from build123d import *

# Parameters (mm, degrees)
SKETCH1_W           = 60.5
SKETCH1_H           = 38.5
BOSS_EXTRUDE1_DEPTH = 6
BOSS_EXTRUDE2_DEPTH = 4
SKETCH4_W           = 6
SKETCH4_H           = 19.5
BOSS_EXTRUDE4_DEPTH = 2
SKETCH6_R           = 2
CUT_EXTRUDE1_DEPTH  = 9
SKETCH7_W           = 48.5
SKETCH7_H           = 2.5
CUT_EXTRUDE2_DEPTH  = 2
CUT_EXTRUDE3_DEPTH  = 4.5
CUT_EXTRUDE4_DEPTH  = 3
SKETCH10_W          = 6
SKETCH10_H          = 7.5
CUT_EXTRUDE5_DEPTH  = 2
SKETCH13_W          = 6
SKETCH13_H          = 10
CUT_EXTRUDE6_DEPTH  = 1.5
CUT_EXTRUDE7_REACH  = 10
SKETCH14_R          = 2


with BuildPart() as part:
    # Sketch1 → Boss-Extrude1 (new body)
    with BuildSketch(Plane(origin=(0, 0, 0), x_dir=(1, 0, 0), z_dir=(0, 1, 0))):
        with Locations((6.235680191, -0.331443914)):
            Rectangle(SKETCH1_W, SKETCH1_H)
    extrude(amount=BOSS_EXTRUDE1_DEPTH)

    # Sketch2 → Boss-Extrude2 (add)
    with BuildSketch(Plane(origin=(0, 6, 0), x_dir=(1, 0, 0), z_dir=(0, 1, 0))):
        Polygon((-24.014319809, -19.581443914), (36.485680191, -19.581443914), (36.485680191, -14.581443914), (36.485680191, -7.081443914), (30.485680191, -7.081443914), (30.485680191, -14.581443914), (-18.014319809, -14.581443914), (-18.014319809, -8.581443914), (-24.014319809, -8.581443914), (-24.014319809, -14.581443914), align=None)
        Polygon((-24.014319809, 18.918556086), (36.485680191, 18.918556086), (36.485680191, 13.918556086), (36.485680191, 6.418556086), (30.485680191, 6.418556086), (30.485680191, 13.918556086), (-24.014319809, 13.918556086), align=None)
    extrude(amount=BOSS_EXTRUDE2_DEPTH)

    # Sketch4 → Boss-Extrude4 (add)
    with BuildSketch(Plane(origin=(0, 6, 0), x_dir=(1, 0, 0), z_dir=(0, 1, 0))):
        with Locations((-21.014319809, 4.168556086)):
            Rectangle(SKETCH4_W, SKETCH4_H)
    extrude(amount=BOSS_EXTRUDE4_DEPTH)

    # Sketch6 → Cut-Extrude1 (cut, through all)
    with BuildSketch(Plane(origin=(0, 8, 0), x_dir=(1, 0, 0), z_dir=(0, 1, 0))):
        with Locations((-21.014319809, -0.331443914)):
            Circle(SKETCH6_R)
    extrude(amount=-CUT_EXTRUDE1_DEPTH, mode=Mode.SUBTRACT)

    # Sketch7 → Cut-Extrude2 (cut)
    with BuildSketch(Plane(origin=(0, 6, 0), x_dir=(1, 0, 0), z_dir=(0, 1, 0))):
        with Locations((6.235680191, 12.668556086)):
            Rectangle(SKETCH7_W, SKETCH7_H)
        with Locations((6.235680191, -13.331443914)):
            Rectangle(SKETCH7_W, SKETCH7_H)
    extrude(amount=-CUT_EXTRUDE2_DEPTH, mode=Mode.SUBTRACT)

    # Sketch8 → Cut-Extrude3 (cut)
    with BuildSketch(Plane(origin=(0, 6, 0), x_dir=(1, 0, 0), z_dir=(0, 1, 0))):
        Polygon((-18.014319809, -5.581443914), (-18.014319809, 9.168556086), (2.985680191, 9.168556086), (2.985680191, -8.581443914), (2.985680191, -9.831443914), (-18.014319809, -9.831443914), (-18.014319809, -8.581443914), (-24.014319809, -8.581443914), (-24.014319809, -5.581443914), align=None)
    extrude(amount=-CUT_EXTRUDE3_DEPTH, mode=Mode.SUBTRACT)

    # Sketch9 → Cut-Extrude4 (cut)
    with BuildSketch(Plane(origin=(0, 6, 0), x_dir=(1, 0, 0), z_dir=(0, 1, 0))):
        Polygon((30.485680191, 9.918556086), (6.485680191, 9.918556086), (6.485680191, -9.581443914), (30.485680191, -9.581443914), (30.485680191, -7.081443914), (36.485680191, -7.081443914), (36.485680191, 6.418556086), (30.485680191, 6.418556086), align=None)
    extrude(amount=-CUT_EXTRUDE4_DEPTH, mode=Mode.SUBTRACT)

    # Sketch10 → Cut-Extrude5 (cut)
    with BuildSketch(Plane(origin=(0, 10, 0), x_dir=(1, 0, 0), z_dir=(0, 1, 0))):
        with Locations((33.485680191, 10.168556086)):
            Rectangle(SKETCH10_W, SKETCH10_H)
        with Locations((33.485680191, -10.831443914)):
            Rectangle(SKETCH10_W, SKETCH10_H)
    extrude(amount=-CUT_EXTRUDE5_DEPTH, mode=Mode.SUBTRACT)

    # Sketch13 → Cut-Extrude6 (cut)
    with BuildSketch(Plane(origin=(0, 3, 0), x_dir=(1, 0, 0), z_dir=(0, 1, 0))):
        with Locations((33.485680191, -0.331443914)):
            Rectangle(SKETCH13_W, SKETCH13_H)
    extrude(amount=-CUT_EXTRUDE6_DEPTH, mode=Mode.SUBTRACT)

    # Sketch14 → Cut-Extrude7 (cut, up to next)
    with BuildSketch(Plane(origin=(0, 8, 0), x_dir=(1, 0, 0), z_dir=(0, 1, 0)), mode=Mode.PRIVATE) as cut_extrude7_sk1:
        with Locations((33.485680191, -10.831443914)):
            Circle(SKETCH14_R)
    cut_extrude7_tool1 = extrude(cut_extrude7_sk1.sketch, amount=-CUT_EXTRUDE7_REACH, mode=Mode.PRIVATE) & part.part
    add(cut_extrude7_tool1.solids().sort_by_distance((33.48568, 8, 10.831444))[0], mode=Mode.SUBTRACT)
    # Sketch14 → Cut-Extrude7 (cut, up to next)
    with BuildSketch(Plane(origin=(0, 8, 0), x_dir=(1, 0, 0), z_dir=(0, 1, 0)), mode=Mode.PRIVATE) as cut_extrude7_sk2:
        with Locations((33.485680191, 10.168556086)):
            Circle(SKETCH14_R)
    cut_extrude7_tool2 = extrude(cut_extrude7_sk2.sketch, amount=-CUT_EXTRUDE7_REACH, mode=Mode.PRIVATE) & part.part
    add(cut_extrude7_tool2.solids().sort_by_distance((33.48568, 8, -10.168556))[0], mode=Mode.SUBTRACT)


solid = part.part
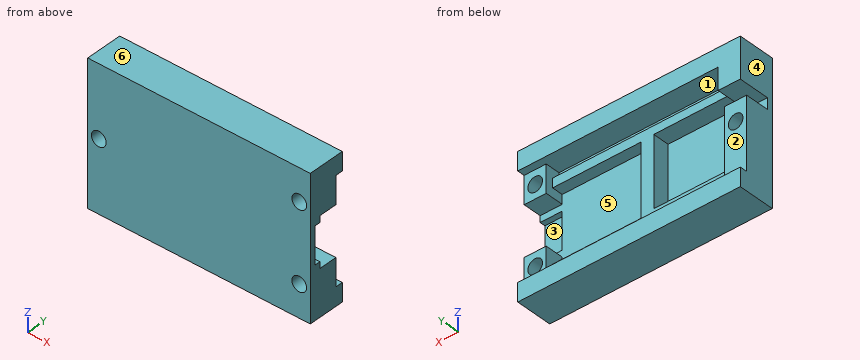
Geometry: final body of the model. Coordinates: model frame, mm. Face numbers are marked on the shaded views. A direction names the side the tool comes from. Round coordinates to 2 decimals unless told otherwise and drop trailing zeros. Write each loop counter-clockwise with the first axis right and the second up, starting at its lowest first coordinate (ties: lowest second). Pieces come first, ordered by that corner, then holes. Notation, with made-up numbers: M -29,-37 L -13,-37 A19 ccw -13,-7 Z; hole C 60.5,39.5 d7. An arc over 180 degrees is marked long. Write item = value, one per line.
Item 1: Pin query (flat end, axial travel): P1, Ø15, axis at x = -15.5, z = 3, coming from the +Y side; P2, Ø6, axis at x = 19, z = -4.5, coming from the +Y side; P3, Ø6, axis at x = -7, z = -2, coming from the +Y side; P4, Ø6.5, axis at x = 33.5, z = 9.5, coming from the +Y side. Return the tip coordinate at first contact, or that it passes through.
Findings:
P1 = 10
P2 = 3
P3 = 1.5
P4 = 8
Item 2: Access query for the marked faces 1, 2 and 3. Directions: +Z, -Z, +X, -X, +Y, -Y. A direction counts if a zero-diameter tool reaches every point of the face in a straight line with its end or side. Return the directions, or none.
Findings:
face_1 = +Y
face_2 = +X, -X, +Y
face_3 = +X, +Y
Item 3: Section query C-C on x = 20.5. Return loops of the section in (y, z).
Findings:
outline = M 0,-18.92 L 10,-18.92 L 10,-13.92 L 4,-13.92 L 4,-11.42 L 6,-11.42 L 6,-9.92 L 3,-9.92 L 3,9.58 L 6,9.58 L 6,12.08 L 4,12.08 L 4,14.58 L 10,14.58 L 10,19.58 L 0,19.58 Z
Item 4: Material intervals for line 1 along Z through (x, y) = (30, 6.5); line 2 along X through (y, z) = (1.5, 11); line 3 along Z through (x, y) = (14, 3.25), sorted ascending. Write a range as [from, to].
Findings:
line_1 = [-18.92, -13.92], [14.58, 19.58]
line_2 = [-24.01, 31.49], [35.48, 36.49]
line_3 = [-18.92, -9.92], [9.58, 19.58]
Item 5: Section query D-D on z = 8. Return loops of the section in (x, y).
Findings:
outline = M -24.01,0 L 36.49,0 L 36.49,8 L 30.49,8 L 30.49,3 L 6.49,3 L 6.49,6 L 2.99,6 L 2.99,1.5 L -24.01,1.5 Z
Item 6: Pull-direction query (X, two-part tool) for the marked faces 4, 5 and 6; classes: pulls with the +X half, pulls with the -X half, needs draft (parallel to the pull), parting line crosses it, or undercut.
Findings:
face_4 = pulls with the -X half
face_5 = undercut
face_6 = needs draft
Item 7: Section query A-A on y = 9. Return loops of the section in (x, z).
Findings:
outline = M -24.01,-18.92 L 36.49,-18.92 L 36.49,-13.92 L -24.01,-13.92 Z; M -24.01,8.58 L -18.01,8.58 L -18.01,14.58 L 36.49,14.58 L 36.49,19.58 L -24.01,19.58 Z
Item 8: Section query B-B on z = -1. Return loops of the section in (x, y).
Findings:
outline = M -24.01,0 L -22.51,0 L -22.51,8 L -24.01,8 Z; M -19.52,0 L 36.49,0 L 36.49,1.5 L 30.49,1.5 L 30.49,3 L 6.49,3 L 6.49,6 L 2.99,6 L 2.99,1.5 L -18.01,1.5 L -18.01,8 L -19.52,8 Z
